Read the model definition and answer for the solid it produces. Units are mm, in the model's axes. Face numbers are marked on the shaded views. A direction names the side the tool comes from. Give positions to 0.01 mm unless a question says otherwise; leave off trailing zeros. Loops run counter-clockwise (first coordinate to the right, second up) from the corner with the lowest first, then second, coordinate; pieces in that order, holes last. Notation, with made-up numbers: (18.5, -37.75) - (65.5, -37.75) arc R19 ccw to (65.5, -12.75) - close; hole circle Ø2 at (36, 52). An arc over 180 degrees is marked (long way). Write item = value, one per line.
```python
from build123d import *

# Parameters (mm, degrees)
F0_R     = 11.5
F1_DEPTH = 20.3
F2_R     = 11.5
F2_R_2   = 9.5
F3_DEPTH = 4
F5_DEPTH = 5
F6_SIZE  = 3
F7_R     = 2
F8_DEPTH = 14.5
F7_R_2   = 8
F9_DEPTH = 3.5


# Not quite as in the source:
# - a fillet or chamfer that OpenCascade refuses, or shapes differently, is made with other operations: its cross-section is extruded or revolved along the edge and cut away or added


with BuildPart() as f1:
    # F0 (on Top) → F1 (new body)
    with BuildSketch(Plane.XY):
        Circle(F0_R)
        with BuildLine():
            ThreePointArc((-7.9375, 0.9980449639), (0, 8), (7.9375, 0.9980449639))
            ThreePointArc((7.9375, 0.9980449639), (8.6846531969, 0.7288689869), (9, 0))
            ThreePointArc((9, 0), (8.6846531969, -0.7288689869), (7.9375, -0.9980449639))
            ThreePointArc((7.9375, -0.9980449639), (0, -8), (-7.9375, -0.9980449639))
            ThreePointArc((-7.9375, -0.9980449639), (-9, 0), (-7.9375, 0.9980449639))
        make_face(mode=Mode.SUBTRACT)
        with BuildLine():
            ThreePointArc((7.9375, 0.9980449639), (7.9843597113, 0.5), (8, 0))
            ThreePointArc((8, 0), (7.9843597113, -0.5), (7.9375, -0.9980449639))
            ThreePointArc((7.9375, -0.9980449639), (8.6846531969, -0.7288689869), (9, 0))
            ThreePointArc((9, 0), (8.6846531969, 0.7288689869), (7.9375, 0.9980449639))
        make_face()
        with BuildLine():
            ThreePointArc((7, 0), (7.2711310131, 0.6846531969), (7.9375, 0.9980449639))
            ThreePointArc((7.9375, 0.9980449639), (0, 8), (-7.9375, 0.9980449639))
            ThreePointArc((-7.9375, 0.9980449639), (-7.2711310131, 0.6846531969), (-7, 0))
            Line((-7, 0), (-6, 0))
            ThreePointArc((-6, 0), (-4.5814370219, 3.8743302407), (-0.9965217286, 5.9166666667))
            ThreePointArc((-0.9965217286, 5.9166666667), (-0.041702946, 6.9991300537), (1, 6))
            ThreePointArc((1, 6), (0.9991300537, 5.958297054), (0.9965217286, 5.9166666667))
            ThreePointArc((0.9965217286, 5.9166666667), (4.5814370219, 3.8743302407), (6, 0))
            Line((6, 0), (7, 0))
        make_face()
        with BuildLine():
            Line((0, 0), (6, 0))
            ThreePointArc((6, 0), (4.5814370219, 3.8743302407), (0.9965217286, 5.9166666667))
            ThreePointArc((0.9965217286, 5.9166666667), (0.6770032004, 5.2640199278), (0, 5))
            Line((0, 5), (0, 0))
        make_face()
        with BuildLine():
            Line((-6, 0), (0, 0))
            Line((0, 0), (0, 5))
            ThreePointArc((0, 5), (-0.6770032004, 5.2640199278), (-0.9965217286, 5.9166666667))
            ThreePointArc((-0.9965217286, 5.9166666667), (-4.5814370219, 3.8743302407), (-6, 0))
        make_face()
        with BuildLine():
            Line((0, -5), (0, 0))
            Line((0, 0), (-6, 0))
            ThreePointArc((-6, 0), (-4.5814370219, -3.8743302407), (-0.9965217286, -5.9166666667))
            ThreePointArc((-0.9965217286, -5.9166666667), (-0.6770032004, -5.2640199278), (0, -5))
        make_face()
        with BuildLine():
            ThreePointArc((0.9965217286, -5.9166666667), (4.5814370219, -3.8743302407), (6, 0))
            Line((6, 0), (0, 0))
            Line((0, 0), (0, -5))
            ThreePointArc((0, -5), (0.6770032004, -5.2640199278), (0.9965217286, -5.9166666667))
        make_face()
        with BuildLine():
            ThreePointArc((0, 5), (0.6770032004, 5.2640199278), (0.9965217286, 5.9166666667))
            ThreePointArc((0.9965217286, 5.9166666667), (0.5, 5.9791303716), (0, 6))
            Line((0, 6), (0, 5))
        make_face()
        with BuildLine():
            Line((0, 5), (0, 6))
            ThreePointArc((0, 6), (-0.5, 5.9791303716), (-0.9965217286, 5.9166666667))
            ThreePointArc((-0.9965217286, 5.9166666667), (-0.6770032004, 5.2640199278), (0, 5))
        make_face()
        with BuildLine():
            ThreePointArc((0, 6), (0.5, 5.9791303716), (0.9965217286, 5.9166666667))
            ThreePointArc((0.9965217286, 5.9166666667), (0.9991300537, 5.958297054), (1, 6))
            ThreePointArc((1, 6), (-0.041702946, 6.9991300537), (-0.9965217286, 5.9166666667))
            ThreePointArc((-0.9965217286, 5.9166666667), (-0.5, 5.9791303716), (0, 6))
        make_face()
        with BuildLine():
            ThreePointArc((7.9375, -0.9980449639), (7.9843597113, -0.5), (8, 0))
            Line((8, 0), (7, 0))
            ThreePointArc((7, 0), (7.2711310131, -0.6846531969), (7.9375, -0.9980449639))
        make_face()
        with BuildLine():
            Line((7, 0), (8, 0))
            ThreePointArc((8, 0), (7.9843597113, 0.5), (7.9375, 0.9980449639))
            ThreePointArc((7.9375, 0.9980449639), (7.2711310131, 0.6846531969), (7, 0))
        make_face()
        with BuildLine():
            ThreePointArc((-7.9375, -0.9980449639), (0, -8), (7.9375, -0.9980449639))
            ThreePointArc((7.9375, -0.9980449639), (7.2711310131, -0.6846531969), (7, 0))
            Line((7, 0), (6, 0))
            ThreePointArc((6, 0), (4.5814370219, -3.8743302407), (0.9965217286, -5.9166666667))
            ThreePointArc((0.9965217286, -5.9166666667), (0.9991300537, -5.958297054), (1, -6))
            ThreePointArc((1, -6), (-0.041702946, -6.9991300537), (-0.9965217286, -5.9166666667))
            ThreePointArc((-0.9965217286, -5.9166666667), (-4.5814370219, -3.8743302407), (-6, 0))
            Line((-6, 0), (-7, 0))
            ThreePointArc((-7, 0), (-7.2711310131, -0.6846531969), (-7.9375, -0.9980449639))
        make_face()
        with BuildLine():
            ThreePointArc((1, -6), (0.9991300537, -5.958297054), (0.9965217286, -5.9166666667))
            ThreePointArc((0.9965217286, -5.9166666667), (0.5, -5.9791303716), (0, -6))
            ThreePointArc((0, -6), (-0.5, -5.9791303716), (-0.9965217286, -5.9166666667))
            ThreePointArc((-0.9965217286, -5.9166666667), (-0.041702946, -6.9991300537), (1, -6))
        make_face()
        with BuildLine():
            ThreePointArc((0, -6), (0.5, -5.9791303716), (0.9965217286, -5.9166666667))
            ThreePointArc((0.9965217286, -5.9166666667), (0.6770032004, -5.2640199278), (0, -5))
            Line((0, -5), (0, -6))
        make_face()
        with BuildLine():
            ThreePointArc((-0.9965217286, -5.9166666667), (-0.5, -5.9791303716), (0, -6))
            Line((0, -6), (0, -5))
            ThreePointArc((0, -5), (-0.6770032004, -5.2640199278), (-0.9965217286, -5.9166666667))
        make_face()
        with BuildLine():
            ThreePointArc((-8, 0), (-7.9843597113, -0.5), (-7.9375, -0.9980449639))
            ThreePointArc((-7.9375, -0.9980449639), (-7.2711310131, -0.6846531969), (-7, 0))
            Line((-7, 0), (-8, 0))
        make_face()
        with BuildLine():
            ThreePointArc((-8, 0), (-7.9843597113, 0.5), (-7.9375, 0.9980449639))
            ThreePointArc((-7.9375, 0.9980449639), (-9, 0), (-7.9375, -0.9980449639))
            ThreePointArc((-7.9375, -0.9980449639), (-7.9843597113, -0.5), (-8, 0))
        make_face()
        with BuildLine():
            ThreePointArc((-7, 0), (-7.2711310131, 0.6846531969), (-7.9375, 0.9980449639))
            ThreePointArc((-7.9375, 0.9980449639), (-7.9843597113, 0.5), (-8, 0))
            Line((-8, 0), (-7, 0))
        make_face()
    extrude(amount=F1_DEPTH)

    # F2 (on face) → F3 (cut)
    with BuildSketch(Plane(origin=(0, 0, 0), x_dir=(1, 0, 0), z_dir=(0, 0, -1))):
        Circle(F2_R)
        Circle(F2_R_2, mode=Mode.SUBTRACT)
    extrude(amount=-F3_DEPTH, mode=Mode.SUBTRACT)

    # F4: fillet of radius 5 on 1 edges, made by hand

    # F4_s1 → F4_t2 (revolve)
    with BuildSketch(Plane.XZ):
        with BuildLine():
            ThreePointArc((11.5, 4), (10.027864045, 2.2360679775), (9.5, 0))
            Line((9.5, 0), (9.5, 4))
            Line((9.5, 4), (11.5, 4))
        make_face()
    revolve(axis=Axis((0, 0, 4), (0, 0, -1)))

    # F0 (on Top) → F5 (cut)
    with BuildSketch(Plane.XY):
        with BuildLine():
            ThreePointArc((-8, 0), (-7.9843597113, 0.5), (-7.9375, 0.9980449639))
            ThreePointArc((-7.9375, 0.9980449639), (-9, 0), (-7.9375, -0.9980449639))
            ThreePointArc((-7.9375, -0.9980449639), (-7.9843597113, -0.5), (-8, 0))
        make_face()
        with BuildLine():
            ThreePointArc((-8, 0), (-7.9843597113, -0.5), (-7.9375, -0.9980449639))
            ThreePointArc((-7.9375, -0.9980449639), (-7.2711310131, -0.6846531969), (-7, 0))
            Line((-7, 0), (-8, 0))
        make_face()
        with BuildLine():
            ThreePointArc((-7, 0), (-7.2711310131, 0.6846531969), (-7.9375, 0.9980449639))
            ThreePointArc((-7.9375, 0.9980449639), (-7.9843597113, 0.5), (-8, 0))
            Line((-8, 0), (-7, 0))
        make_face()
        with BuildLine():
            ThreePointArc((0, 6), (0.5, 5.9791303716), (0.9965217286, 5.9166666667))
            ThreePointArc((0.9965217286, 5.9166666667), (0.9991300537, 5.958297054), (1, 6))
            ThreePointArc((1, 6), (-0.041702946, 6.9991300537), (-0.9965217286, 5.9166666667))
            ThreePointArc((-0.9965217286, 5.9166666667), (-0.5, 5.9791303716), (0, 6))
        make_face()
        with BuildLine():
            ThreePointArc((0, 5), (0.6770032004, 5.2640199278), (0.9965217286, 5.9166666667))
            ThreePointArc((0.9965217286, 5.9166666667), (0.5, 5.9791303716), (0, 6))
            Line((0, 6), (0, 5))
        make_face()
        with BuildLine():
            Line((0, 5), (0, 6))
            ThreePointArc((0, 6), (-0.5, 5.9791303716), (-0.9965217286, 5.9166666667))
            ThreePointArc((-0.9965217286, 5.9166666667), (-0.6770032004, 5.2640199278), (0, 5))
        make_face()
        with BuildLine():
            ThreePointArc((7.9375, 0.9980449639), (7.9843597113, 0.5), (8, 0))
            ThreePointArc((8, 0), (7.9843597113, -0.5), (7.9375, -0.9980449639))
            ThreePointArc((7.9375, -0.9980449639), (8.6846531969, -0.7288689869), (9, 0))
            ThreePointArc((9, 0), (8.6846531969, 0.7288689869), (7.9375, 0.9980449639))
        make_face()
        with BuildLine():
            ThreePointArc((7.9375, -0.9980449639), (7.9843597113, -0.5), (8, 0))
            Line((8, 0), (7, 0))
            ThreePointArc((7, 0), (7.2711310131, -0.6846531969), (7.9375, -0.9980449639))
        make_face()
        with BuildLine():
            Line((7, 0), (8, 0))
            ThreePointArc((8, 0), (7.9843597113, 0.5), (7.9375, 0.9980449639))
            ThreePointArc((7.9375, 0.9980449639), (7.2711310131, 0.6846531969), (7, 0))
        make_face()
        with BuildLine():
            ThreePointArc((1, -6), (0.9991300537, -5.958297054), (0.9965217286, -5.9166666667))
            ThreePointArc((0.9965217286, -5.9166666667), (0.5, -5.9791303716), (0, -6))
            ThreePointArc((0, -6), (-0.5, -5.9791303716), (-0.9965217286, -5.9166666667))
            ThreePointArc((-0.9965217286, -5.9166666667), (-0.041702946, -6.9991300537), (1, -6))
        make_face()
        with BuildLine():
            ThreePointArc((-0.9965217286, -5.9166666667), (-0.5, -5.9791303716), (0, -6))
            Line((0, -6), (0, -5))
            ThreePointArc((0, -5), (-0.6770032004, -5.2640199278), (-0.9965217286, -5.9166666667))
        make_face()
        with BuildLine():
            ThreePointArc((0, -6), (0.5, -5.9791303716), (0.9965217286, -5.9166666667))
            ThreePointArc((0.9965217286, -5.9166666667), (0.6770032004, -5.2640199278), (0, -5))
            Line((0, -5), (0, -6))
        make_face()
    extrude(amount=F5_DEPTH, mode=Mode.SUBTRACT)

    # F6
    f6_edges = [f1.edges().sort_by_distance(p)[0] for p in [
        (-11.5, 0, 20.3),
    ]]
    chamfer(f6_edges, length=F6_SIZE)

    # F7 (on face) → F8 (join)
    with BuildSketch(Plane.XY.offset(20.3)):
        Circle(F7_R)
    extrude(amount=F8_DEPTH)

    # F7 (on face) → F9 (join)
    with BuildSketch(Plane.XY.offset(20.3)):
        Circle(F7_R_2)
        Circle(F7_R, mode=Mode.SUBTRACT)
    extrude(amount=F9_DEPTH)


solid = f1.part
```
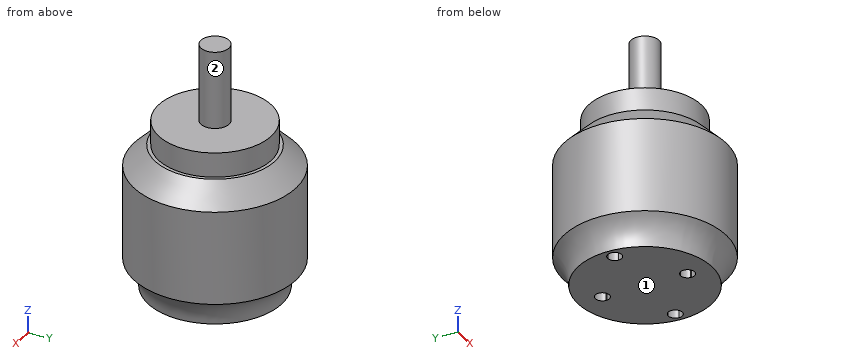
1) A cutting plane is placed at B-B on z = 28. Determine the outline of the cut face in (x, y), then the cut area to 3 significant figures.
Output:
outline = circle Ø4 at (0, 0)
area = 12.6 mm²
2) A cutting plane is placed at A-A on z = 3.5. Determine the outline of the cut face in (x, y).
Output:
outline = circle Ø21.86 at (0, 0); hole circle Ø2 at (-8, 0); hole circle Ø2 at (0, -6); hole circle Ø2 at (0, 6); hole circle Ø2 at (8, 0)
3) Find the intervals of material crossed by probe 1 along Z at (x, y) = (-2.75, 2.25); probe 2 along Z at (x, y) = (5.5, -6.25); probe 3 along X at (y, z) = (2.5, 10), in increasing order.
Output:
probe_1 = 0 to 23.8
probe_2 = 0 to 20.3
probe_3 = -11.22 to 11.22
4) A cutting plane is placed at C-C on z = 19.5. Determine the outline of the cut face in (x, y), then the cut area to 3 significant figures.
Output:
outline = circle Ø18.6 at (0, 0)
area = 272 mm²
5) Each of these flat-tipped pins is pushed along its axis until it touches: P1, Ø1, axis at x = 0.5, y = -5.5, coming from the -Z side; P2, Ø8, axis at x = -4.5, z = 27, coming from the +Y side; P3, Ø12, axis at y = 7.5, z = 10, coming from the -X side; P4, Ø6, axis at x = -1, z = 26.5, coming from the -Y side. Where does it stop, or does it pass through?
Output:
P1 = 0
P2 = 7.72
P3 = -11.4
P4 = -8
6) A tool of negligible diameter and unlimited length cuts with its end or side. For the marked faces 1 and 2, from which of +Z, -Z, +X, -X, +Y, -Y can it reach the whole face along a straight path? Write none if from no direction.
Output:
face_1 = -Z, +X, -X, +Y, -Y
face_2 = +Z
